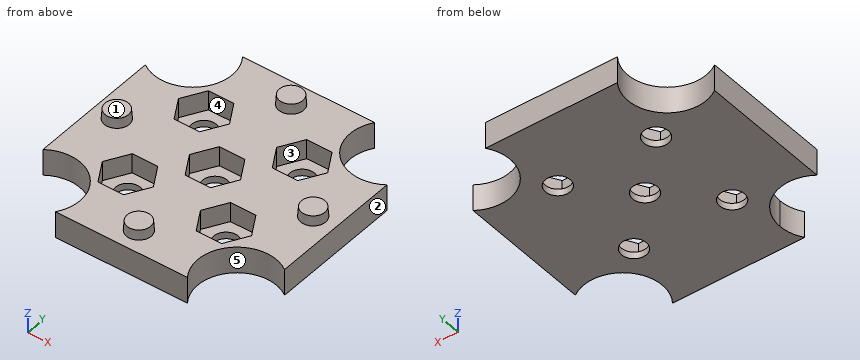
from build123d import *

# Parameters (mm, degrees)
F0_R       = 3.2004
F0_R_2     = 6.858
F1_DEPTH   = 6.8326
F2_DEPTH   = 9.3726
F3_R       = 3.2004
F4_DEPTH   = 5.08
F5_SIZE2   = 2.53999
F5_SIZE    = 0.17779
F5_2_SIZE2 = 2.53999
F5_2_SIZE  = 0.17779
F5_3_SIZE2 = 2.53999
F5_3_SIZE  = 0.17779
F5_4_SIZE2 = 2.53999
F5_4_SIZE  = 0.17779


# Not quite as in the source:
# - a fillet or chamfer is up to 0.001 mm smaller than in the source, because OpenCascade refuses the exact size


with BuildPart() as f1:
    # F0 (on Top) → F1 (new body)
    with BuildSketch(Plane.XY):
        with BuildLine():
            ThreePointArc((-31.242, -17.0875613686), (-20.7164714157, -16.3838944106), (-15.24, -25.4))
            ThreePointArc((-15.24, -25.4), (-15.712895776, -28.4635945803), (-17.0875613686, -31.242))
            Line((-17.0875613686, -31.242), (17.0875613686, -31.242))
            ThreePointArc((17.0875613686, -31.242), (18.2157951031, -18.2157951031), (31.242, -17.0875613686))
            Line((31.242, -17.0875613686), (31.242, 17.0875613686))
            ThreePointArc((31.242, 17.0875613686), (18.2157951031, 18.2157951031), (17.0875613686, 31.242))
            Line((17.0875613686, 31.242), (-17.0875613686, 31.242))
            ThreePointArc((-17.0875613686, 31.242), (-18.2157951031, 18.2157951031), (-31.242, 17.0875613686))
            Line((-31.242, 17.0875613686), (-31.242, -17.0875613686))
        make_face()
        with Locations((0, -25.4)):
            Circle(F0_R, mode=Mode.SUBTRACT)
        with Locations((-25.4, 0)):
            Circle(F0_R, mode=Mode.SUBTRACT)
        with Locations((-12.7, -12.7)):
            Circle(F0_R, mode=Mode.SUBTRACT)
        Circle(F0_R_2, mode=Mode.SUBTRACT)
        with Locations((12.7, -12.7)):
            Circle(F0_R, mode=Mode.SUBTRACT)
        with Locations((25.4, 0)):
            Circle(F0_R, mode=Mode.SUBTRACT)
        with Locations((-12.7, 12.7)):
            Circle(F0_R, mode=Mode.SUBTRACT)
        with Locations((0, 25.4)):
            Circle(F0_R, mode=Mode.SUBTRACT)
        with Locations((12.7, 12.7)):
            Circle(F0_R, mode=Mode.SUBTRACT)
        Circle(F0_R_2)
        Circle(F0_R, mode=Mode.SUBTRACT)
    extrude(amount=F1_DEPTH)

    # F0 (on Top) → F2 (join)
    with BuildSketch(Plane.XY):
        with Locations((-25.4, 0)):
            Circle(F0_R)
        with Locations((0, -25.4)):
            Circle(F0_R)
        with Locations((25.4, 0)):
            Circle(F0_R)
        with Locations((0, 25.4)):
            Circle(F0_R)
    extrude(amount=F2_DEPTH)

    # F3 (on face) → F4 (cut)
    with BuildSketch(Plane.XY.offset(6.8326)):
        Polygon((-9.398, 6.9807682334), (-6.096, 12.7), (-9.398, 18.4192317666), (-16.002, 18.4192317666), (-19.304, 12.7), (-16.002, 6.9807682334), align=None)
        with Locations((-12.7, 12.7)):
            Circle(F3_R, mode=Mode.SUBTRACT)
        Polygon((9.398, 18.4192317666), (6.096, 12.7), (9.398, 6.9807682334), (16.002, 6.9807682334), (19.304, 12.7), (16.002, 18.4192317666), align=None)
        with Locations((12.7, 12.7)):
            Circle(F3_R, mode=Mode.SUBTRACT)
        Polygon((-9.398, -18.4192317666), (-6.096, -12.7), (-9.398, -6.9807682334), (-16.002, -6.9807682334), (-19.304, -12.7), (-16.002, -18.4192317666), align=None)
        with Locations((-12.7, -12.7)):
            Circle(F3_R, mode=Mode.SUBTRACT)
        Polygon((9.398, -6.9807682334), (6.096, -12.7), (9.398, -18.4192317666), (16.002, -18.4192317666), (19.304, -12.7), (16.002, -6.9807682334), align=None)
        with Locations((12.7, -12.7)):
            Circle(F3_R, mode=Mode.SUBTRACT)
        Polygon((3.302, -5.7192317666), (6.604, 0), (3.302, 5.7192317666), (-3.302, 5.7192317666), (-6.604, 0), (-3.302, -5.7192317666), align=None)
        Circle(F3_R, mode=Mode.SUBTRACT)
    extrude(amount=-F4_DEPTH, mode=Mode.SUBTRACT)

    # F5 (size 0.1778 and 2.54 in the source; OpenCascade refuses exactly that, so slightly less here)
    f5_edges = [f1.edges().sort_by_distance(p)[0] for p in [
        (-28.6004, 0, 9.3726),
    ]]
    f5_side = f1.faces().sort_by_distance((-25.4, 0, 9.3726))[0]
    chamfer(f5_edges, length=F5_SIZE, length2=F5_SIZE2, reference=f5_side)

    # F5#2 (size 0.1778 and 2.54 in the source; OpenCascade refuses exactly that, so slightly less here)
    f5_2_edges = [f1.edges().sort_by_distance(p)[0] for p in [
        (-3.2004, 25.4, 9.3726),
    ]]
    f5_2_side = f1.faces().sort_by_distance((0, 25.4, 9.3726))[0]
    chamfer(f5_2_edges, length=F5_2_SIZE, length2=F5_2_SIZE2, reference=f5_2_side)

    # F5#3 (size 0.1778 and 2.54 in the source; OpenCascade refuses exactly that, so slightly less here)
    f5_3_edges = [f1.edges().sort_by_distance(p)[0] for p in [
        (22.1996, 0, 9.3726),
    ]]
    f5_3_side = f1.faces().sort_by_distance((25.4, 0, 9.3726))[0]
    chamfer(f5_3_edges, length=F5_3_SIZE, length2=F5_3_SIZE2, reference=f5_3_side)

    # F5#4 (size 0.1778 and 2.54 in the source; OpenCascade refuses exactly that, so slightly less here)
    f5_4_edges = [f1.edges().sort_by_distance(p)[0] for p in [
        (-3.2004, -25.4, 9.3726),
    ]]
    f5_4_side = f1.faces().sort_by_distance((0, -25.4, 9.3726))[0]
    chamfer(f5_4_edges, length=F5_4_SIZE, length2=F5_4_SIZE2, reference=f5_4_side)


solid = f1.part
For this review, take the finished solid that the model builds, in its own axes (mm). Face numbers are marked on the shaded views. A direction names the side the tool comes from. Coordinates: 2 decimals unless noted, no trailing zeros. Loops run counter-clockwise (first coordinate to the right, second up) from the corner with the lowest first, then second, coordinate; pieces in that order, holes last. Notation, with made-up numbers: (-1.75, 29.5) - (44.25, 29.5) arc R15 ccw to (44.25, 55.5) - close; hole circle Ø4 at (8, -2.75). An arc over 180 degrees is marked (long way). Use a Markdown table: item, result. Add a question column.
Item 1: We need section D-D (x = -8.5). Give the boundary of the cut face in (y, z).
Item 2: Mouldability with a two-part tool opening along X and no side actions: class the marked faces 1, 2 and 3 as pulls with the +X half, pulls with the -X half, needs draft (parallel to the pull), parting line crosses it, or undercut.
Item 3: We need section C-C (z = 5.25). Give the number of separate pieces and of enclosed holes in the cut face, and give its area (3 significant figures).
Item 4: Tool access review of the marked faces 4 and 5: name each direction out of +Z, -Z, +X, -X, +Y, -Y from which nothing blocks a thin tool from reaching the whole face with its end or side.
Item 5: For line 1 (Y direction, x = -12.7, z = 0.9); line 2 (Y direction, x = 13.5, z = 5); line 3 (Y direction, x = 0, z = 0.65), list the stretches that pass through material, from the lowest coordinate up.
Item 6: Insertion check: pin 1 Ø5.5 at (x, y) = (-15, 14) entering from +Z; pin 2 Ø12.5 at (x, y) = (-2, 2.5) entering from +Z. Each pin has a flat end and moves straight along its axis. Give the tip position at first contact, or say it passes through.
Item 7: We need section A-A (x = 12.7). Give the boundary of the cut face in (y, z), and give its area (3 significant figures).
Results list:
| question | item | result |
|---|---|---|
| 1 | outline | (-31.24, 0) - (31.24, 0) - (31.24, 6.83) - (16.86, 6.83) - (16.86, 1.75) - (8.54, 1.75) - (8.54, 6.83) - (-8.54, 6.83) - (-8.54, 1.75) - (-16.86, 1.75) - (-16.86, 6.83) - (-31.24, 6.83) - close |
| 2 | face 1 | needs draft |
| 2 | face 2 | pulls with the +X half |
| 2 | face 3 | undercut |
| 3 | separate pieces | 1 |
| 3 | enclosed holes | 5 |
| 3 | area | 2,430 mm^2 |
| 4 | face 4 | +Z |
| 4 | face 5 | +Z, -Z |
| 5 | line 1 | y = -31.24 to -15.9, -9.5 to 9.5, 15.9 to 31.24 |
| 5 | line 2 | y = -31.24 to -18.42, -6.98 to 6.98, 18.42 to 31.24 |
| 5 | line 3 | y = -31.24 to -3.2, 3.2 to 31.24 |
| 6 | pin 1 | stops at z = 1.75 |
| 6 | pin 2 | stops at z = 6.83 |
| 7 | outline | (-31.24, 0) - (-15.9, 0) - (-15.9, 1.75) - (-18.42, 1.75) - (-18.42, 6.83) - (-31.24, 6.83) - close; (-9.5, 0) - (9.5, 0) - (9.5, 1.75) - (6.98, 1.75) - (6.98, 6.83) - (-6.98, 6.83) - (-6.98, 1.75) - (-9.5, 1.75) - close; (15.9, 0) - (31.24, 0) - (31.24, 6.83) - (18.42, 6.83) - (18.42, 1.75) - (15.9, 1.75) - close |
| 7 | area | 288 mm^2 |
